The model under review builds one solid part; all positions refer to its coordinate system, in mm. Coordinates: 2 decimals unless noted, no trailing zeros. Write each loop counter-clockwise with the first axis right and the second up, starting at its lowest first coordinate (ties: lowest second). Pieces come first, ordered by that corner, then holes. Notation, with made-up numbers: (41.5, 12.5) - (64.5, 12.5) arc R16 cw to (64.5, 33.5) - close; hole circle Ø9 at (-16, 0.25). An arc over 180 degrees is marked (long way). Put each result on its own line as item: value.
from build123d import *

# Parameters (mm, degrees)
ESQUISSE1_R             = 10
BOSS_EXTRU_1_DEPTH      = 2
CONG_1_R                = 0.25
ENL_V_MAT_EXTRU_1_DEPTH = 0.25


with BuildPart() as part:
    # Esquisse1 → Boss.-Extru.1 (new body)
    with BuildSketch(Plane.XY):
        Circle(ESQUISSE1_R)
    extrude(amount=BOSS_EXTRU_1_DEPTH)

    # Congé1
    cong_1_edges = [part.edges().sort_by_distance(p)[0] for p in [
        (-10, 0, 0),
        (-10, 0, 2),
    ]]
    fillet(cong_1_edges, radius=CONG_1_R)

    # Esquisse2 → Enlèv. mat.-Extru.1 (cut)
    with BuildSketch(Plane(origin=(0, 0, 0), x_dir=(-1, 0, 0), z_dir=(0, 0, -1))):
        with BuildLine():
            Line((-1.923076923, -1.852508928), (-1.415865385, -1.54842239))
            add(Edge.make_bspline(
                [(-1.415865385, -1.54842239), (-1.368691264, -1.627389907), (-1.278307468, -1.778688622), (-1.12753371, -1.983130977), (-0.971305862, -2.156894674), (-0.808467004, -2.298968859), (-0.640011093, -2.410824093), (-0.46483843, -2.490027919), (-0.283539326, -2.539426734), (-0.160155632, -2.545426882), (-0.098557692, -2.54842239)],
                knots=[0, 0, 0, 0, 1.272034388, 2.437168799, 3.508375237, 4.49857839, 5.41946034, 6.295179144, 7.148887113, 8, 8, 8, 8], degree=3))
            add(Edge.make_bspline(
                [(-0.098557692, -2.54842239), (-0.045951646, -2.546957237), (0.058339965, -2.544052568), (0.211875239, -2.516142621), (0.3609869, -2.473264686), (0.502601707, -2.411857375), (0.634765618, -2.337562828), (0.75066281, -2.247826524), (0.850856147, -2.147358742), (0.932814629, -2.035274192), (0.99569469, -1.914730508), (1.04402395, -1.791000306), (1.070844076, -1.662139903), (1.074884225, -1.57537911), (1.076923077, -1.531595467)],
                knots=[0, 0, 0, 0, 1.095163259, 2.171163733, 3.241058638, 4.321873601, 5.38011039, 6.391990106, 7.366004449, 8.327778327, 9.272591725, 10.192022065, 11.087607919, 12, 12, 12, 12], degree=3))
            add(Edge.make_bspline(
                [(1.076923077, -1.531595467), (1.074395687, -1.481639724), (1.069257873, -1.380087), (1.025832479, -1.230259023), (0.957519484, -1.081986046), (0.894497809, -0.990269591), (0.861778846, -0.942653159)],
                knots=[0, 0, 0, 0, 0.938893495, 1.908633276, 2.914225137, 4, 4, 4, 4], degree=3))
            add(Edge.make_bspline(
                [(0.861778846, -0.942653159), (0.834914936, -0.908287176), (0.778517517, -0.836140092), (0.681561781, -0.72874826), (0.5677913, -0.617973828), (0.441099491, -0.499586873), (0.296871339, -0.379093507), (0.139624172, -0.250747888), (-0.03465673, -0.119430899), (-0.156884438, -0.031363643), (-0.219951923, 0.01407761)],
                knots=[0, 0, 0, 0, 0.722233717, 1.516239348, 2.393582979, 3.351407094, 4.387010283, 5.505090956, 6.712668013, 8, 8, 8, 8], degree=3))
            add(Edge.make_bspline(
                [(-0.219951923, 0.01407761), (-0.283078774, 0.059040903), (-0.403772505, 0.145007296), (-0.572558646, 0.272591783), (-0.723492011, 0.389238416), (-0.855901754, 0.496045294), (-0.969729634, 0.593026902), (-1.065872625, 0.679251941), (-1.14188158, 0.757052331), (-1.184148289, 0.807523202), (-1.203125, 0.83018338)],
                knots=[0, 0, 0, 0, 1.452282411, 2.77665338, 3.964542531, 5.026858415, 5.96415736, 6.766646006, 7.446254459, 8, 8, 8, 8], degree=3))
            add(Edge.make_bspline(
                [(-1.203125, 0.83018338), (-1.229649363, 0.865499443), (-1.281813083, 0.934953221), (-1.350669093, 1.04351012), (-1.409193372, 1.154635718), (-1.455071655, 1.268628628), (-1.493705173, 1.383888506), (-1.519690198, 1.501919213), (-1.535961164, 1.622191131), (-1.537627426, 1.70312856), (-1.538461538, 1.743644918)],
                knots=[0, 0, 0, 0, 1.068054152, 2.10047183, 3.106115577, 4.101338837, 5.06977816, 6.043150881, 7.020423561, 8, 8, 8, 8], degree=3))
            add(Edge.make_bspline(
                [(-1.538461538, 1.743644918), (-1.536224037, 1.807124532), (-1.53179686, 1.932726927), (-1.494355973, 2.11620835), (-1.435259584, 2.291385065), (-1.352468348, 2.45652278), (-1.245741457, 2.607321605), (-1.122234073, 2.745516154), (-0.975128668, 2.861690866), (-0.813724171, 2.963197252), (-0.637056104, 3.04264741), (-0.451928841, 3.102580518), (-0.258048146, 3.136539246), (-0.126728487, 3.141412557), (-0.060096154, 3.143885303)],
                knots=[0, 0, 0, 0, 1.005424448, 1.989358655, 2.955360095, 3.929531133, 4.905563448, 5.876582895, 6.856512386, 7.866279853, 8.892233794, 9.918561126, 10.94386622, 12, 12, 12, 12], degree=3))
            add(Edge.make_bspline(
                [(-0.060096154, 3.143885303), (0.010608018, 3.141446643), (0.15121605, 3.136596927), (0.358043276, 3.09442973), (0.557175933, 3.02465715), (0.717364387, 2.945476593), (0.842734835, 2.866394166), (0.938345234, 2.794360182), (1.035232293, 2.711431424), (1.134177529, 2.617387002), (1.233504374, 2.511364001), (1.334687435, 2.394088534), (1.437963325, 2.266277295), (1.504401942, 2.175035294), (1.538461538, 2.128260303)],
                knots=[0, 0, 0, 0, 1.286793592, 2.559021753, 3.825965368, 5.121522368, 5.803751409, 6.523245864, 7.299691795, 8.125521123, 9.008227632, 9.944561021, 10.946284179, 12, 12, 12, 12], degree=3))
            Line((1.538461538, 2.128260303), (1.051682692, 1.759269918))
            add(Edge.make_bspline(
                [(1.051682692, 1.759269918), (1.022289665, 1.797136244), (0.965685567, 1.870057936), (0.879749304, 1.972180191), (0.798751622, 2.065465585), (0.718950937, 2.146491518), (0.644561854, 2.219695175), (0.57236121, 2.282369044), (0.503388037, 2.335127208), (0.416444761, 2.391430454), (0.307214387, 2.447241602), (0.170098039, 2.494468593), (0.026807282, 2.5228487), (-0.070786372, 2.526601078), (-0.120192308, 2.528500687)],
                knots=[0, 0, 0, 0, 1.181633172, 2.275549214, 3.290209073, 4.226197932, 5.078386478, 5.862611352, 6.581680152, 7.217281963, 8.414376989, 9.595101626, 10.782541182, 12, 12, 12, 12], degree=3))
            add(Edge.make_bspline(
                [(-0.120192308, 2.528500687), (-0.182174918, 2.526423487), (-0.301702542, 2.522417803), (-0.471400089, 2.478669257), (-0.624132532, 2.409786068), (-0.755365501, 2.313246105), (-0.86462889, 2.198867261), (-0.943666819, 2.067246366), (-0.99123853, 1.921905105), (-0.997043581, 1.820519408), (-1, 1.768885303)],
                knots=[0, 0, 0, 0, 1.14458467, 2.207223713, 3.21896685, 4.227309161, 5.202851033, 6.127160689, 7.046193047, 8, 8, 8, 8], degree=3))
            add(Edge.make_bspline(
                [(-1, 1.768885303), (-0.999326069, 1.736739911), (-0.997977104, 1.672396563), (-0.979163165, 1.577336983), (-0.954992887, 1.482517544), (-0.916691232, 1.388364545), (-0.863813569, 1.293231358), (-0.794376125, 1.195479808), (-0.706924732, 1.094248307), (-0.639935568, 1.028407095), (-0.604567308, 0.993644918)],
                knots=[0, 0, 0, 0, 0.858281714, 1.717966888, 2.583508476, 3.4729293, 4.427298488, 5.488583878, 6.674047936, 8, 8, 8, 8], degree=3))
            add(Edge.make_bspline(
                [(-0.604567308, 0.993644918), (-0.591433526, 0.981924302), (-0.560230668, 0.954078802), (-0.503186224, 0.908492036), (-0.427855713, 0.852258712), (-0.336206225, 0.782680455), (-0.226547891, 0.701969377), (-0.098868652, 0.61115747), (0.045408262, 0.507296683), (0.147788689, 0.434683757), (0.201923077, 0.396289149)],
                knots=[0, 0, 0, 0, 0.420754252, 0.999615792, 1.744751191, 2.668019286, 3.750313428, 4.999500688, 6.413464383, 8, 8, 8, 8], degree=3))
            add(Edge.make_bspline(
                [(0.201923077, 0.396289149), (0.267041785, 0.348903961), (0.393135139, 0.257149112), (0.572548133, 0.119293661), (0.735223233, -0.015531085), (0.881731582, -0.146464126), (1.013520568, -0.272512285), (1.129128089, -0.395192023), (1.229732112, -0.513624434), (1.338039344, -0.665463135), (1.448709892, -0.851944993), (1.543752476, -1.080421974), (1.603681072, -1.309787095), (1.611517955, -1.463947386), (1.615384615, -1.540008928)],
                knots=[0, 0, 0, 0, 1.163667725, 2.253281268, 3.268753668, 4.215851969, 5.092017293, 5.902905408, 6.650798638, 7.335211899, 8.59617414, 9.77448103, 10.901945474, 12, 12, 12, 12], degree=3))
            add(Edge.make_bspline(
                [(1.615384615, -1.540008928), (1.614258093, -1.593800411), (1.612026924, -1.700338783), (1.586379643, -1.856776058), (1.548803075, -2.008714691), (1.492167816, -2.154276598), (1.423042402, -2.296124763), (1.335328834, -2.430538307), (1.233658518, -2.560492133), (1.117029206, -2.682520975), (0.98940766, -2.794543025), (0.854521326, -2.894192845), (0.712149429, -2.977281399), (0.563064315, -3.045082843), (0.407231738, -3.09811173), (0.244704109, -3.136533791), (0.075213518, -3.16011501), (-0.039987308, -3.162562601), (-0.098557692, -3.163807005)],
                knots=[0, 0, 0, 0, 0.983748083, 1.948392443, 2.894712957, 3.844097841, 4.80183111, 5.778335162, 6.776009319, 7.81870978, 8.863265674, 9.881300176, 10.883814829, 11.87499822, 12.874611388, 13.892143829, 14.928324115, 16, 16, 16, 16], degree=3))
            add(Edge.make_bspline(
                [(-0.098557692, -3.163807005), (-0.143875423, -3.162930694), (-0.233940155, -3.161189107), (-0.367156409, -3.145792627), (-0.497681419, -3.12400902), (-0.623877331, -3.089424901), (-0.747370037, -3.047464368), (-0.867622439, -2.995798655), (-0.984692817, -2.933883453), (-1.099237245, -2.863091982), (-1.210964401, -2.780707277), (-1.318826346, -2.684752712), (-1.426362093, -2.577874703), (-1.53039763, -2.45717088), (-1.633037305, -2.32459131), (-1.732257436, -2.178895567), (-1.830111809, -2.020877246), (-1.891509754, -1.909679956), (-1.923076923, -1.852508928)],
                knots=[0, 0, 0, 0, 0.915332311, 1.819136955, 2.706846663, 3.586547465, 4.459518054, 5.340707479, 6.227863349, 7.133153174, 8.059268498, 9.028702269, 10.047606654, 11.120612155, 12.245963614, 13.433783089, 14.680604001, 16, 16, 16, 16], degree=3))
        make_face()
    extrude(amount=-ENL_V_MAT_EXTRU_1_DEPTH, mode=Mode.SUBTRACT)


solid = part.part
1. Consider section A-A on z = 1.05. State the section outline as (x, y) points.
Determined:
outline: circle Ø20 at (0, 0)
2. The part is to be moulded in two halves that separate along Y. For faces 1 (the cylindrical face through (-2.17, -9.76, 0.99)), 2 (the flat face through (0, 0.2, 0.25)), 3 (the flat face through (0, -2, 0)), say which applies: +Y half, -Y half, draft (parallel to the pull), parting line (faces both ways), or undercut.
Determined:
face 1: parting line
face 2: undercut
face 3: draft
3. To check wall thickness, follow probe 1 along Y at (x, z) = (0.25, 1.55); probe 2 along Z at (x, y) = (1, -2.5); probe 3 along Y at (x, z) = (2.75, 1.45). State the ranges of each line that lie inside material, in increasing order.
Determined:
probe 1: y = -10 to 10
probe 2: z = 0.25 to 2
probe 3: y = -9.61 to 9.61
